Here's how the part is built. I have some questions about the finished solid (model axes, mm). Give positions to 0.01 mm unless a question says otherwise; leave off trailing zeros. Loops run counter-clockwise (first coordinate to the right, second up) from the corner with the lowest first, then second, coordinate; pieces in that order, holes last. Notation, with made-up numbers: (-34, 53) - (0, 53) arc R21 cw to (0, 84) - close; hole circle Ø11 at (-28.5, -20.75). An arc over 180 degrees is marked (long way). Use a Markdown table: item, result.
from build123d import *

# Parameters (mm, degrees)
SKETCH1_W           = 11
SKETCH1_H           = 35
BOSS_EXTRUDE1_DEPTH = 3
SKETCH2_R           = 1.5
CUT_EXTRUDE1_DEPTH  = 3
FILLET1_R           = 3
SKETCH3_W           = 1.5
SKETCH3_H           = 10
BOSS_EXTRUDE2_DEPTH = 0.5
FILLET4_R           = 2
FILLET5_R           = 0.5


with BuildPart() as part:
    # Sketch1 → Boss-Extrude1 (new body)
    with BuildSketch(Plane(origin=(0, 0, 0), x_dir=(1, 0, 0), z_dir=(0, 1, 0))):
        Rectangle(SKETCH1_W, SKETCH1_H)
    extrude(amount=BOSS_EXTRUDE1_DEPTH)

    # Sketch2 → Cut-Extrude1 (cut)
    with BuildSketch(Plane(origin=(0, 3, 0), x_dir=(1, 0, 0), z_dir=(0, 1, 0))):
        with Locations(Location((3, 15, 0), (0, 0, 270))):
            Circle(SKETCH2_R)
    extrude(amount=-CUT_EXTRUDE1_DEPTH, mode=Mode.SUBTRACT)

    # Fillet1
    fillet1_edges = [part.edges().sort_by_distance(p)[0] for p in [
        (-5.5, 1.5, -17.5),
    ]]
    fillet(fillet1_edges, radius=FILLET1_R)

    # Sketch3 → Boss-Extrude2 (add)
    with BuildSketch(Plane(origin=(0, 3, 0), x_dir=(1, 0, 0), z_dir=(0, 1, 0))):
        with Locations((-1.167481663, -10)):
            Rectangle(SKETCH3_W, SKETCH3_H)
        with Locations((-3.667481663, -10)):
            Rectangle(SKETCH3_W, SKETCH3_H)
        with Locations((1.332518337, -10)):
            Rectangle(SKETCH3_W, SKETCH3_H)
        with Locations((3.832518337, -10)):
            Rectangle(SKETCH3_W, SKETCH3_H)
    extrude(amount=BOSS_EXTRUDE2_DEPTH)

    # Fillet4
    fillet4_edges = [part.edges().sort_by_distance(p)[0] for p in [
        (0, 3, 17.5),
    ]]
    fillet(fillet4_edges, radius=FILLET4_R)

    # Fillet5
    fillet5_edges = [part.edges().sort_by_distance(p)[0] for p in [
        (5.5, 1.5, -17.5),
        (5.5, 3, -1),
        (5.5, 0.5, 17.5),
        (5.5, 2.414213562, 16.914213562),
    ]]
    fillet(fillet5_edges, radius=FILLET5_R)


solid = part.part
(1) If I drill on line 1 (X direction, y = 3.25, z = 12); line 2 (Y direction, x = -2.75, z = -6); line 3 (X direction, y = 1.35, z = -15), over which ranges is the centre line in solid material (lowest first)?
A:
| item | result |
|---|---|
| line 1 | -4.42 to -2.92, -1.92 to -0.42, 0.58 to 2.08, 3.08 to 4.58 |
| line 2 | 0 to 3 |
| line 3 | -5.46 to 1.5, 4.5 to 5.5 |
(2) Suppose I cut it at A-A on x = 1. Write out the boundary of the cut face in (y, z), plus the area to 3 significant figures.
A:
| item | result |
|---|---|
| outline | (0, -17.5) - (3, -17.5) - (3, 5) - (3.5, 5) - (3.5, 15) - (3, 15) - (3, 15.5) arc R2 ccw to (1, 17.5) - (0, 17.5) - close |
| area | 109 mm2 |
(3) We'd pull the mould along X, two halves only. Please class faces 1 (the face through (-0.18, 2.4, 16.93)), 2 (the face through (3.07, 1.52, -16.5)), 3 (the face through (5.5, 1, 0)), 4 (the face through (-4.64, 1.52, -16.6)): pulls with the +X half, pulls with the -X half, needs draft (parallel to the pull), parting line crosses it, or undercut.
A:
| item | result |
|---|---|
| face 1 | needs draft |
| face 2 | undercut |
| face 3 | pulls with the +X half |
| face 4 | pulls with the -X half |
(4) Will these pins go through, and if not, where does the flat tip stop? pin 1 (0.6 mm diameter, centred on y = 3.5, z = 11.5, fed in from -X); pin 2 (4 mm diameter, centred on x = -2, z = -9, fed in from +Y); pin 3 (0.6 mm diameter, centred on y = 3, z = 7.5, fed in from +X).
A:
| item | result |
|---|---|
| pin 1 | x = -4.42 |
| pin 2 | y = 3 |
| pin 3 | x = 5.46 |
(5) Suppose I cut it at B-B on z = -15. Write out the boundary of the cut face in (x, y).
A:
| item | result |
|---|---|
| outline | (-5.46, 0) - (1.5, 0) - (1.5, 3) - (-5.46, 3) - close; (4.5, 0) - (5.5, 0) - (5.5, 2.5) arc R0.5 ccw to (5, 3) - (4.5, 3) - close |
(6) Suppose I cut it at C-C on z = -7. Write out the boundary of the cut face in (x, y), plus the area to 3 significant figures.
A:
| item | result |
|---|---|
| outline | (-5.5, 0) - (5.5, 0) - (5.5, 2.5) arc R0.5 ccw to (5, 3) - (-5.5, 3) - close |
| area | 32.9 mm2 |
